```python
from build123d import *

# Parameters (mm, degrees)
F0_R     = 1.75
F1_DEPTH = 2.5
F3_DEPTH = 0.8
F4_SIZE  = 0.5


with BuildPart() as f1:
    # F0 (on Top) → F1 (new body)
    with BuildSketch(Plane.XY):
        with BuildLine():
            ThreePointArc((2.984962, 14.7), (0, 18), (-2.984962, 14.7))
            ThreePointArc((-2.984962, 14.7), (0, -15), (2.984962, 14.7))
        make_face()
        with Locations((0, 15)):
            Circle(F0_R, mode=Mode.SUBTRACT)
    extrude(amount=F1_DEPTH)

    # F2 (on face) → F3 (join)
    with BuildSketch(Plane.XY.offset(2.5)):
        with BuildLine():
            Line((-4.133975, 1.886751), (4.133975, 1.886751))
            ThreePointArc((4.133975, 1.886751), (4.566987, 2.136751), (4.566987, 2.636751))
            Line((4.566987, 2.636751), (0.433013, 9.797005))
            ThreePointArc((0.433013, 9.797005), (0, 10.047005), (-0.433013, 9.797005))
            Line((-0.433013, 9.797005), (-4.566987, 2.636751))
            ThreePointArc((-4.566987, 2.636751), (-4.566987, 2.136751), (-4.133975, 1.886751))
        make_face()
        with BuildLine():
            ThreePointArc((-4.566987, 1.136751), (-5, 1.386751), (-5.433013, 1.136751))
            Line((-5.433013, 1.136751), (-9.566987, -6.023503))
            ThreePointArc((-9.566987, -6.023503), (-9.566987, -6.523503), (-9.133975, -6.773503))
            Line((-9.133975, -6.773503), (-0.866025, -6.773503))
            ThreePointArc((-0.866025, -6.773503), (-0.433013, -6.523503), (-0.433013, -6.023503))
            Line((-0.433013, -6.023503), (-4.566987, 1.136751))
        make_face()
        with BuildLine():
            Line((4.566987, 1.136751), (0.433013, -6.023503))
            ThreePointArc((0.433013, -6.023503), (0.433013, -6.523503), (0.866025, -6.773503))
            Line((0.866025, -6.773503), (9.133975, -6.773503))
            ThreePointArc((9.133975, -6.773503), (9.566987, -6.523503), (9.566987, -6.023503))
            Line((9.566987, -6.023503), (5.433013, 1.136751))
            ThreePointArc((5.433013, 1.136751), (5, 1.386751), (4.566987, 1.136751))
        make_face()
    extrude(amount=F3_DEPTH)

    # F4
    f4_edges = [f1.edges().sort_by_distance(p)[0] for p in [
        (0, -15, 2.5),
        (0, -15, 0),
        (0, 18, 2.5),
        (0, 18, 0),
        (-1.75, 15, 0),
        (-1.75, 15, 2.5),
    ]]
    chamfer(f4_edges, length=F4_SIZE)


solid = f1.part
```
Geometry: final body of the model. Coordinates: model frame, mm. A direction names the side the tool comes from. Coordinates: 2 decimals unless noted, no trailing zeros. Order: outer loops, then holes, each group sorted by start corner. A loop starts at its lowest first (then second) coordinate and runs counter-clockwise, first axis right, second up. Notation, with made-up numbers: (-37, -12.75) -> (-29, -12.75) arc R32 ccw to (-29, 26.25) -> close; hole circle Ø9 at (-26.5, -22.5). An arc over 180 degrees is marked (long way). Answer in a Markdown table with one row per item.
Item 1: Section A-A on x = 0. Output: boundary loops of the cut face in (y, z), plus the area to 3 significant figures.
Return value:
| item | result |
|---|---|
| outline | (-15, 0.5) -> (-14.5, 0) -> (12.75, 0) -> (13.25, 0.5) -> (13.25, 2) -> (12.75, 2.5) -> (10.05, 2.5) -> (10.05, 3.3) -> (1.89, 3.3) -> (1.89, 2.5) -> (-14.5, 2.5) -> (-15, 2) -> close; (16.75, 0.5) -> (17.25, 0) -> (17.5, 0) -> (18, 0.5) -> (18, 2) -> (17.5, 2.5) -> (17.25, 2.5) -> (16.75, 2) -> close |
| area | 79.3 mm² |
Item 2: Section B-B on y = 0. Output: boundary loops of the cut face in (x, z).
Return value:
| item | result |
|---|---|
| outline | (-15, 0.5) -> (-14.5, 0) -> (14.5, 0) -> (15, 0.5) -> (15, 2) -> (14.5, 2.5) -> (6.09, 2.5) -> (6.09, 3.3) -> (3.91, 3.3) -> (3.91, 2.5) -> (-3.91, 2.5) -> (-3.91, 3.3) -> (-6.09, 3.3) -> (-6.09, 2.5) -> (-14.5, 2.5) -> (-15, 2) -> close |
Item 3: Contact query for flat-ended pins moving along their axis: P1, Ø1.5, axis at x = -10, y = -8, coming from the +Z side; P2, Ø0.9, axis at x = 6.5, z = 3, coming from the -Y side; P3, Ø1.5, axis at x = 3, z = 2, coming from the +Y side. Output: stop coordinate, or through.
Return value:
| item | result |
|---|---|
| P1 | stops at z = 2.5 |
| P2 | stops at y = -6.77 |
| P3 | stops at y = 16.98 |
Item 4: Ray query, L1, parallel to Z at x = -5, y = -10.5; L2, parallel to Y at x = 3.5, z = 2.95; L3, parallel to X at y = -2, z = 2.3. Return the intervals inside material, ascending.
Return value:
| item | result |
|---|---|
| L1 | z = 0 to 2.5 |
| L2 | y = -6.77 to -0.71, 1.89 to 4.48 |
| L3 | x = -14.56 to 14.56 |
Item 5: Section C-C on z = 0.9. Output: boundary loops of the cut face in (x, y), plus the area to 3 significant figures.
Return value:
| item | result |
|---|---|
| outline | (-2.98, 14.7) arc R15 ccw (long way) to (2.98, 14.7) arc R3 ccw (long way) to start; hole circle Ø3.5 at (0, 15) |
| area | 712 mm² |
Item 6: Access query for faces 1 (the flat face through (-2.471, -2.493, 2.894)), 2 (the flat face through (-7.47, -2.39, 2.89)), 3 (the flat face through (7.529, -2.493, 2.894)). Directions: +Z, -Z, +X, -X, +Y, -Y. A direction counts if a zero-diameter tool reaches every point of the face in a straight line with its end or side. Return the directions, or none.
Return value:
| item | result |
|---|---|
| face 1 | +Z |
| face 2 | +Z, -X, +Y |
| face 3 | +Z, +X, +Y |
Item 7: Draft query along Y for faces 4 (the flat face through (-2.47, 6.27, 2.89)), 5 (the flat face through (2.53, -2.39, 2.89)), 6 (the flat face through (-5, -4, 3.3)), 7 (the cylindrical face through (-0.228, 16.735, 1.24)). Return one class per face: released by +Y, released by -Y, zero draft, split by the parting line, or undercut.
Return value:
| item | result |
|---|---|
| face 4 | released by +Y |
| face 5 | undercut |
| face 6 | zero draft |
| face 7 | undercut |
